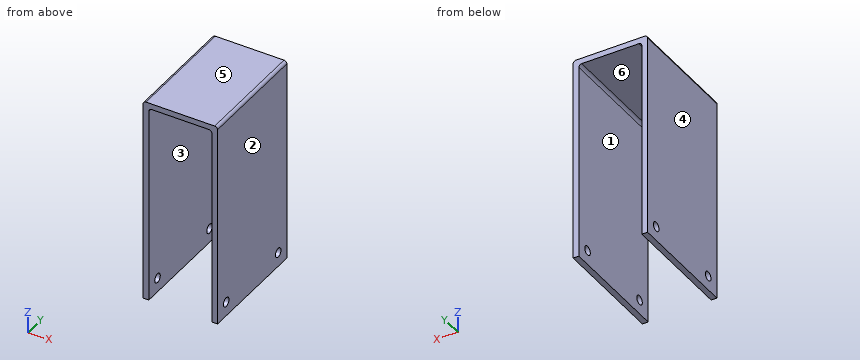
from build123d import *

# Parameters (mm, degrees)
F1_DEPTH = 200
F2_R     = 5
F3_R     = 8
F4_DEPTH = 400


with BuildPart() as f1:
    # F0 (on Front) → F1 (new body)
    with BuildSketch(Plane.XZ):
        Polygon((0, 360), (0, 0), (10, 0), (10, 350), (120, 350), (120, 0), (130, 0), (130, 360), align=None)
    extrude(amount=F1_DEPTH)

    # F2
    f2_edges = [f1.edges().sort_by_distance(p)[0] for p in [
        (130, -100, 360),
        (0, -100, 360),
        (10, -100, 350),
        (120, -100, 350),
    ]]
    fillet(f2_edges, radius=F2_R)

    # F3 (on face) → F4 (cut)
    with BuildSketch(Plane.YZ.offset(130)):
        with Locations((-25, 25)):
            Circle(F3_R)
        with Locations((-175, 25)):
            Circle(F3_R)
    extrude(amount=-F4_DEPTH, mode=Mode.SUBTRACT)


solid = f1.part
The listing builds one solid part. Answer for the finished solid, in the listing's coordinates (mm). Face numbers are marked on the shaded views. A direction names the side the tool comes from. Coordinates: 2 decimals unless noted, no trailing zeros. Write each loop counter-clockwise with the first axis right and the second up, starting at its lowest first coordinate (ties: lowest second). Pieces come first, ordered by that corner, then holes. Notation, with made-up numbers: (-40, 68.5) - (-23, 68.5) arc R26 cw to (-23, 82.5) - close; hole circle Ø8 at (-3, 87). An arc over 180 degrees is marked (long way). Put each result on its own line as item: value.
1. The part is cut by section C-C on z = 162. Give the vertices of the cut face in (x, y).
Answer sheet:
outline: (0, -200) - (10, -200) - (10, 0) - (0, 0) - close; (120, -200) - (130, -200) - (130, 0) - (120, 0) - close
2. Find the intervals of material crossed by line 1 along X through (y, z) = (-56, 19); line 2 along Z through (x, y) = (123.5, -25); line 3 along Z through (x, y) = (21, -30.5), in increasing order. Write a range as from..to.
Answer sheet:
line 1: x = 0..10, 120..130
line 2: z = 0..17, 33..360
line 3: z = 350..360
3. The part is cut by section B-B on z = 25. Give the vertices of the cut face in (x, y), plus the area to 3 significant figures.
Answer sheet:
outline: (0, -200) - (10, -200) - (10, -183) - (0, -183) - close; (0, -167) - (10, -167) - (10, -33) - (0, -33) - close; (0, -17) - (10, -17) - (10, 0) - (0, 0) - close; (120, -200) - (130, -200) - (130, -183) - (120, -183) - close; (120, -167) - (130, -167) - (130, -33) - (120, -33) - close; (120, -17) - (130, -17) - (130, 0) - (120, 0) - close
area: 3,360 mm^2
4. Flat-ended cylindrical pins translate along their axes: pin 1 Ø9.5 at (y, z) = (-175, 25) entering from -X (3 decimals); pin 2 Ø2 at (x, y) = (92.5, -81) entering from -Z. Find the tip coordinate at first contact, or state that the pin passes through.
Answer sheet:
pin 1: passes through
pin 2: stops at z = 350
5. A tool of negligible diameter and unlimited length cuts with its end or side. For the marked faces 1 and 2, from which of +Z, -Z, +X, -X, +Y, -Y can it reach the whole face along a straight path? Write none if from no direction.
Answer sheet:
face 1: -Z, +Y, -Y
face 2: +Z, -Z, +X, +Y, -Y
6. The part is cut by section D-D on y = -58.5. Give the vertices of the cut face in (x, z), plus the area to 3 significant figures.
Answer sheet:
outline: (0, 0) - (10, 0) - (10, 345) arc R5 cw to (15, 350) - (115, 350) arc R5 cw to (120, 345) - (120, 0) - (130, 0) - (130, 355) arc R5 ccw to (125, 360) - (5, 360) arc R5 ccw to (0, 355) - close
area: 8,300 mm^2
7. Determine the mould class of the marked faces 3, 4, 5 and 6 for opening direction X: pulls with the +X half, pulls with the -X half, needs draft (parallel to the pull), parting line crosses it, or undercut.
Answer sheet:
face 3: undercut
face 4: pulls with the -X half
face 5: needs draft
face 6: undercut
8. The part is cut by section A-A on y = -175. Give the vertices of the cut face in (x, z).
Answer sheet:
outline: (0, 0) - (10, 0) - (10, 17) - (0, 17) - close; (0, 33) - (10, 33) - (10, 345) arc R5 cw to (15, 350) - (115, 350) arc R5 cw to (120, 345) - (120, 33) - (130, 33) - (130, 355) arc R5 ccw to (125, 360) - (5, 360) arc R5 ccw to (0, 355) - close; (120, 0) - (130, 0) - (130, 17) - (120, 17) - close
